Design review of the part shown in the three views and the two pictorial views. Dimensions are in mm from the part's minimum x, y and z. A direction names the side the tool comes from. Coordinates: 2 decimals unless noted, no trailing zeros. Order: outer loops, then holes, each group sorted by start corner. A loop starts at its lowest first (then second) coordinate and runs counter-clockwise, first axis right, second up. Notation, with made-up numbers: (38.25, -8) -> (80.25, -8) arc R14 cw to (80.25, 2) -> close; hole circle Ø4 at (-16, 3.5). An arc over 180 degrees is marked (long way). Write item = value, one per line. Start each with the question number.
1) Insertion check: pin 1 Ø4 at (x, z) = (1190, 315) entering from +Y; pin 2 Ø6 at (x, y) = (1550.5, 825) entering from +Z. Each pin has a flat end and moves straight along its axis. Give the tip position at first contact, or say it passes through.
2) Consider section A-A on x = 735. Give the boundary of the cut face in (y, z).
3) Wall thickness on probe 1 along Z at (x, y) = (618, 771); probe 2 along Y at (x, z) = (494.5, 324): over which ranges is each line inside the solid? List them lowest first. Write a range as [from, to].
4) Machinability: for the marked faces 1 and 2, which of the approach directions +Z, -Z, +X, -X, +Y, -Y give a long, thin tool a straight path to every point of the face, cutting with its end or side? Answer none if there is none.
5) Consider section B-B on z = 577. Give the boundary of the cut face in (x, y), and give its area (3 significant figures).
6) Consider section C-C on y = 677. Give the boundary of the cut face in (x, z).
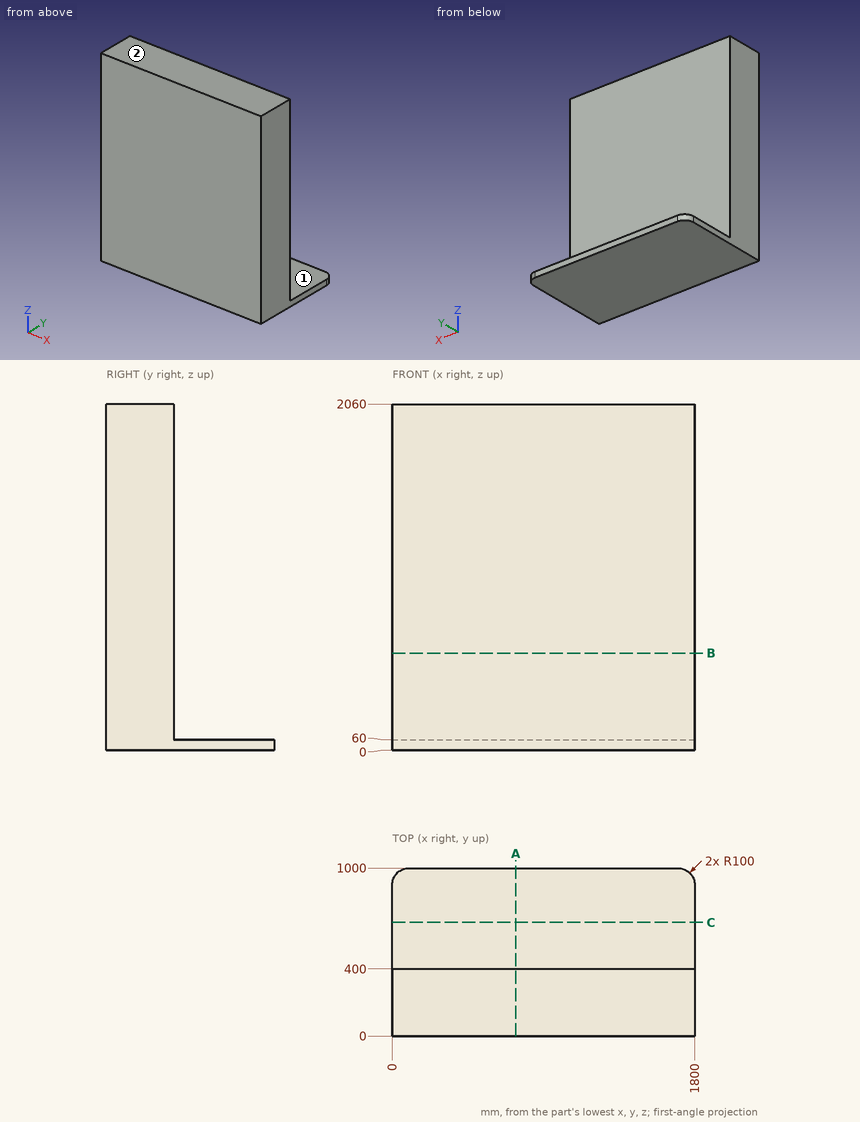
Answer sheet:
q1.pin_1 = 400
q1.pin_2 = 60
q2.outline = (0, 0) -> (1000, 0) -> (1000, 60) -> (400, 60) -> (400, 2060) -> (0, 2060) -> close
q3.probe_1 = [0, 60]
q3.probe_2 = [0, 400]
q4.face_1 = +Z, +X, -X, +Y
q4.face_2 = +Z, +X, -X, +Y, -Y
q5.outline = (0, 0) -> (1800, 0) -> (1800, 400) -> (0, 400) -> close
q5.area = 720,000 mm2
q6.outline = (0, 0) -> (1800, 0) -> (1800, 60) -> (0, 60) -> close
